from build123d import *

# Parameters (mm, degrees)
SKIZZE1_W                       = 25
SKIZZE1_H                       = 31.5
AUFSATZ_LINEAR_AUSTRAGEN1_DEPTH = 2
SKIZZE2_W                       = 22
SKIZZE2_H                       = 29
AUFSATZ_LINEAR_AUSTRAGEN2_DEPTH = 16.5
SKIZZE3_W                       = 1
SKIZZE3_H                       = 25
AUFSATZ_LINEAR_AUSTRAGEN3_DEPTH = 6
SKIZZE4_W                       = 5
SKIZZE4_H                       = 1
AUFSATZ_LINEAR_AUSTRAGEN4_DEPTH = 7
SKIZZE5_W                       = 18
SKIZZE5_H                       = 24
AUFSATZ_LINEAR_AUSTRAGEN5_DEPTH = 4
SKIZZE6_R                       = 37
SCHNITT_LINEAR_AUSTRAGEN1_DEPTH = 36.532555495


with BuildPart() as part:
    # Skizze1 → Aufsatz-Linear austragen1 (new body)
    with BuildSketch(Plane(origin=(0, 0, 0), x_dir=(1, 0, 0), z_dir=(0, 1, 0))):
        Rectangle(SKIZZE1_W, SKIZZE1_H)
    extrude(amount=AUFSATZ_LINEAR_AUSTRAGEN1_DEPTH)

    # Skizze2 → Aufsatz-Linear austragen2 (add)
    with BuildSketch(Plane.XZ):
        Rectangle(SKIZZE2_W, SKIZZE2_H)
    extrude(amount=AUFSATZ_LINEAR_AUSTRAGEN2_DEPTH)

    # Skizze3 → Aufsatz-Linear austragen3 (add)
    with BuildSketch(Plane.XZ.offset(16.5)):
        Rectangle(SKIZZE3_W, SKIZZE3_H)
    extrude(amount=AUFSATZ_LINEAR_AUSTRAGEN3_DEPTH)

    # Skizze4 → Aufsatz-Linear austragen4 (add)
    with BuildSketch(Plane.XZ.offset(16.5)):
        with Locations((-5, 9.5)):
            Rectangle(SKIZZE4_W, SKIZZE4_H)
        with Locations((-5, 0)):
            Rectangle(SKIZZE4_W, SKIZZE4_H)
        with Locations((-5, -9.5)):
            Rectangle(SKIZZE4_W, SKIZZE4_H)
        with Locations((5, -9.5)):
            Rectangle(SKIZZE4_W, SKIZZE4_H)
        with Locations((5, 0)):
            Rectangle(SKIZZE4_W, SKIZZE4_H)
        with Locations((5, 9.5)):
            Rectangle(SKIZZE4_W, SKIZZE4_H)
    extrude(amount=AUFSATZ_LINEAR_AUSTRAGEN4_DEPTH)

    # Skizze5 → Aufsatz-Linear austragen5 (add)
    with BuildSketch(Plane(origin=(0, 2, 0), x_dir=(1, 0, 0), z_dir=(0, 1, 0))):
        Rectangle(SKIZZE5_W, SKIZZE5_H)
    extrude(amount=AUFSATZ_LINEAR_AUSTRAGEN5_DEPTH)

    # Skizze6 → Schnitt-Linear austragen1 (cut, through all)
    with BuildSketch(Plane.ZY.offset(9)):
        with Locations((0, 41)):
            Circle(SKIZZE6_R)
    extrude(amount=-SCHNITT_LINEAR_AUSTRAGEN1_DEPTH, mode=Mode.SUBTRACT)


solid = part.part
Read the model definition and answer for the solid it produces. Units are mm, in the model's axes. A direction names the side the tool comes from. Give positions to 0.01 mm unless a question says otherwise; leave off trailing zeros. Loops run counter-clockwise (first coordinate to the right, second up) from the corner with the lowest first, then second, coordinate; pieces in that order, holes last. Notation, with made-up numbers: (57.25, -11) -> (66.25, -11) arc R22 cw to (66.25, 9) -> close; hole circle Ø8 at (74.5, -1). An arc over 180 degrees is marked (long way). Answer as CSV lines item,"result".
Item 1: Find section A-A on y = -21.5. Give the vertices of the cut face in (x, z).
Returned:
outline,"(-7.5, -10) -> (-2.5, -10) -> (-2.5, -9) -> (-7.5, -9) -> close; (-7.5, -0.5) -> (-2.5, -0.5) -> (-2.5, 0.5) -> (-7.5, 0.5) -> close; (-7.5, 9) -> (-2.5, 9) -> (-2.5, 10) -> (-7.5, 10) -> close; (-0.5, -12.5) -> (0.5, -12.5) -> (0.5, 12.5) -> (-0.5, 12.5) -> close; (2.5, -10) -> (7.5, -10) -> (7.5, -9) -> (2.5, -9) -> close; (2.5, -0.5) -> (7.5, -0.5) -> (7.5, 0.5) -> (2.5, 0.5) -> close; (2.5, 9) -> (7.5, 9) -> (7.5, 10) -> (2.5, 10) -> close"
Item 2: Find section D-D on x = 1.25. Give the vertices of the cut face in (y, z).
Returned:
outline,"(-16.5, -14.5) -> (0, -14.5) -> (0, -15.75) -> (2, -15.75) -> (2, -12) -> (6, -12) arc R37 cw to (6, 12) -> (2, 12) -> (2, 15.75) -> (0, 15.75) -> (0, 14.5) -> (-16.5, 14.5) -> close"
Item 3: Each of these flat-tipped pins is pushed along its axis until it touches: pin 1 (1.5 mm diameter, centred on x = -5.5, y = -20, fed in from -Z); pin 2 (0.8 mm diameter, centred on y = -18.5, z = 0, fed in from +X); pin 3 (3 mm diameter, centred on x = 8.5, z = 6.5, fed in from -Y). Where does it stop, or does it pass through?
Returned:
pin 1,"stops at z = -10"
pin 2,"stops at x = 7.5"
pin 3,"stops at y = -16.5"
Item 4: For faces 4 (the face through (5, -20, -0.5)), 5 (the face through (-2.5, -20, 0)), 6 (the face through (-7.5, -20, -9.5)), determine the directions among +Z, -Z, +X, -X, +Y, -Y from which every point of the face is accessible in a straight line to the end or side of a thin tool.
Returned:
face 4,"+X, -Y"
face 5,"+Z, -Z, -Y"
face 6,"+Z, -Z, -X, -Y"
Item 5: Find section C-C on z = 13. Give the vertices of the cut face in (x, y).
Returned:
outline,"(-12.5, 0) -> (-11, 0) -> (-11, -16.5) -> (11, -16.5) -> (11, 0) -> (12.5, 0) -> (12.5, 2) -> (-12.5, 2) -> close"
Item 6: Determine the mould class of faces 1 (the face through (5, -20, -10)), 2 (the face through (2.5, -20, 0)), 3 (the face through (-12.5, 1, 0)) for opening direction X: +X half, -X half, draft (parallel to the pull), parting line (faces both ways), or undercut.
Returned:
face 1,"draft"
face 2,"undercut"
face 3,"-X half"
Item 7: Consider line 1 (Z direction, x = 6.25, y = -19); line 2 (Z direction, x = 6.75, y = -9.5); line 3 (Y direction, x = 9.25, z = 0). Determine where each line is inside the solid, lowest interval first. Write a range as [from, to].
Returned:
line 1,"z = [-10, -9], [-0.5, 0.5], [9, 10]"
line 2,"z = [-14.5, 14.5]"
line 3,"y = [-16.5, 2]"
Item 8: Find section B-B on x = -3. Give the vertices of the cut face in (y, z).
Returned:
outline,"(-23.5, -10) -> (-16.5, -10) -> (-16.5, -14.5) -> (0, -14.5) -> (0, -15.75) -> (2, -15.75) -> (2, -12) -> (6, -12) arc R37 cw to (6, 12) -> (2, 12) -> (2, 15.75) -> (0, 15.75) -> (0, 14.5) -> (-16.5, 14.5) -> (-16.5, 10) -> (-23.5, 10) -> (-23.5, 9) -> (-16.5, 9) -> (-16.5, 0.5) -> (-23.5, 0.5) -> (-23.5, -0.5) -> (-16.5, -0.5) -> (-16.5, -9) -> (-23.5, -9) -> close"
